Geometry: see drawing. Coordinates: mm, zero at the bounding-box minimum. A direction names the side the tool comes from. Coordinates: 2 decimals unless noted, no trailing zeros. Loops run counter-clockwise (first coordinate to the right, second up) from the corner with the lowest first, then second, coordinate; pieces in that order, holes last. Notation, with made-up numbers: (39.5, -20) -> (66.5, -20) arc R12 cw to (66.5, -4) -> close; hole circle Ø2 at (75.25, 61). An arc over 180 degrees is marked (long way). One line per item, written item: value. Start each with the question number.
Item 1: Set-up query: the marked faces 1 and 2. Return all of +Z, -Z, +X, -X, +Y, -Y with unobstructed straight access to the full face (end or side cutting, diameter ignored); none if empty.
Item 2: Section query C-C on x = 33.5. Return loops of the section in (y, z).
Item 3: Section query A-A on z = 21.15. Return loops of the section in (x, y).
Item 4: Section query D-D on z = 32. Return loops of the section in (x, y).
Item 5: Contact query for a flat-ended pin moving along its axis: pin 1 Ø12 at (x, z) = (7, 14.5) entering from +Y. Output: stop coordinate, or through.
Item 6: Section query B-B on x = 21.15. Return loops of the section in (y, z).
Item 7: Ray query, probe 1 along Y at (x, z) = (35.5, 29.5); probe 2 along X at (y, z) = (50, 22). Return the intervals inside material, ascending. Write a range as from..to.
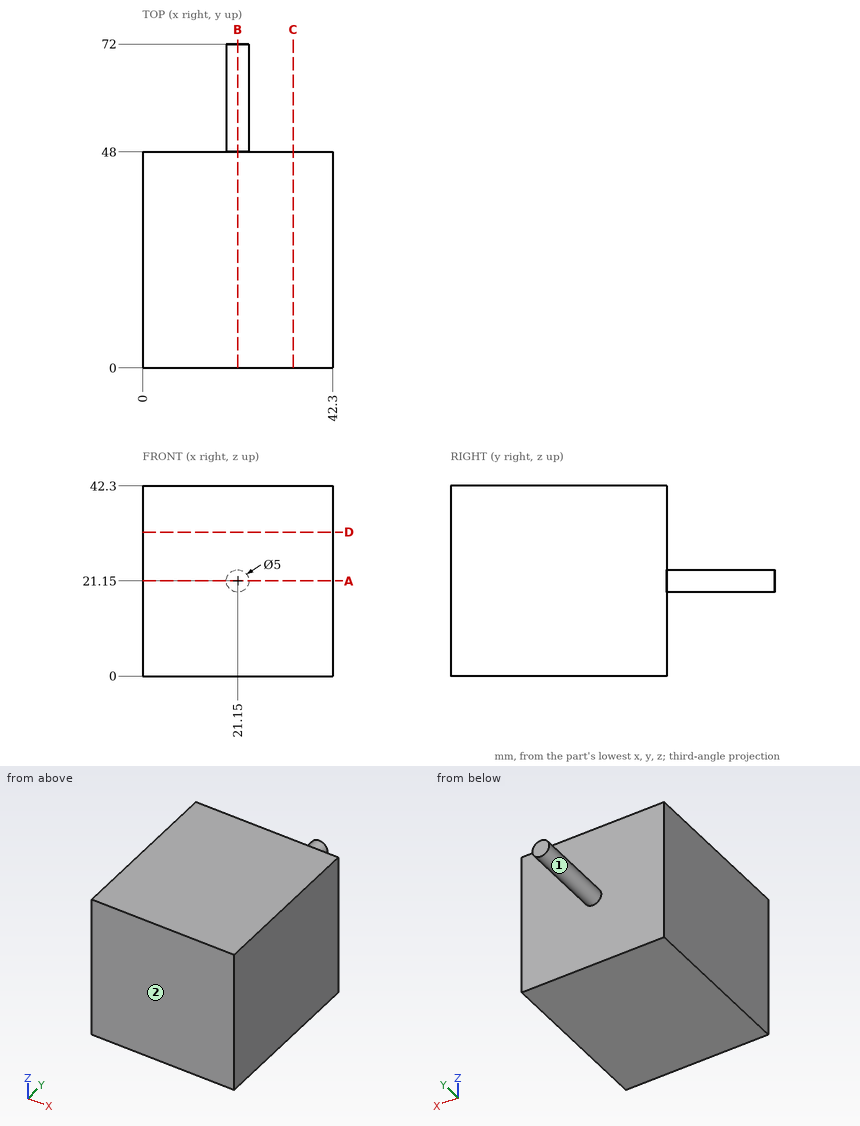
Reply:
1. face 1: +Y
1. face 2: +Z, -Z, +X, -X, -Y
2. outline: (0, 0) -> (48, 0) -> (48, 42.3) -> (0, 42.3) -> close
3. outline: (0, 0) -> (42.3, 0) -> (42.3, 48) -> (23.65, 48) -> (23.65, 72) -> (18.65, 72) -> (18.65, 48) -> (0, 48) -> close
4. outline: (0, 0) -> (42.3, 0) -> (42.3, 48) -> (0, 48) -> close
5. pin 1: stops at y = 48
6. outline: (0, 0) -> (48, 0) -> (48, 18.65) -> (72, 18.65) -> (72, 23.65) -> (48, 23.65) -> (48, 42.3) -> (0, 42.3) -> close
7. probe 1: y = 0..48
7. probe 2: x = 18.8..23.5
